Check sheet for the drawn part. Datum: minimum x, y, z corner. Units: mm. Coordinates: 2 decimals unless noted, no trailing zeros. Write each loop counter-clockwise with the first axis right and the second up, starting at its lowest first coordinate (ties: lowest second). Pieces come first, ordered by that corner, then holes. Notation, with made-up numbers: (20, 13) -> (50, 13) arc R28 ccw to (50, 50) -> close; hole circle Ø8 at (2, 29.5). An arc over 180 degrees is marked (long way). Answer in a Markdown table with one row per item. Add a question column.
1. Scan lines: L1, parallel to X at y = 1.05, z = 3.1; L2, parallel to Z at x = 54.9, y = 1.45; L3, parallel to X at y = 1.75, z = 29. Record each from-to range of solid material in increasing order. Write a range as from..to.
2. Cross-section at B-B on x = 54.9. Record the cut outline in (y, z), and give its area (3 significant figures).
3. Cross-section at A-A on z = 3.1. Record the cut outline in (x, y), and give its area (3 significant figures).
4. Cross-section at C-C on y = 1.3. Record the cut outline in (x, z).
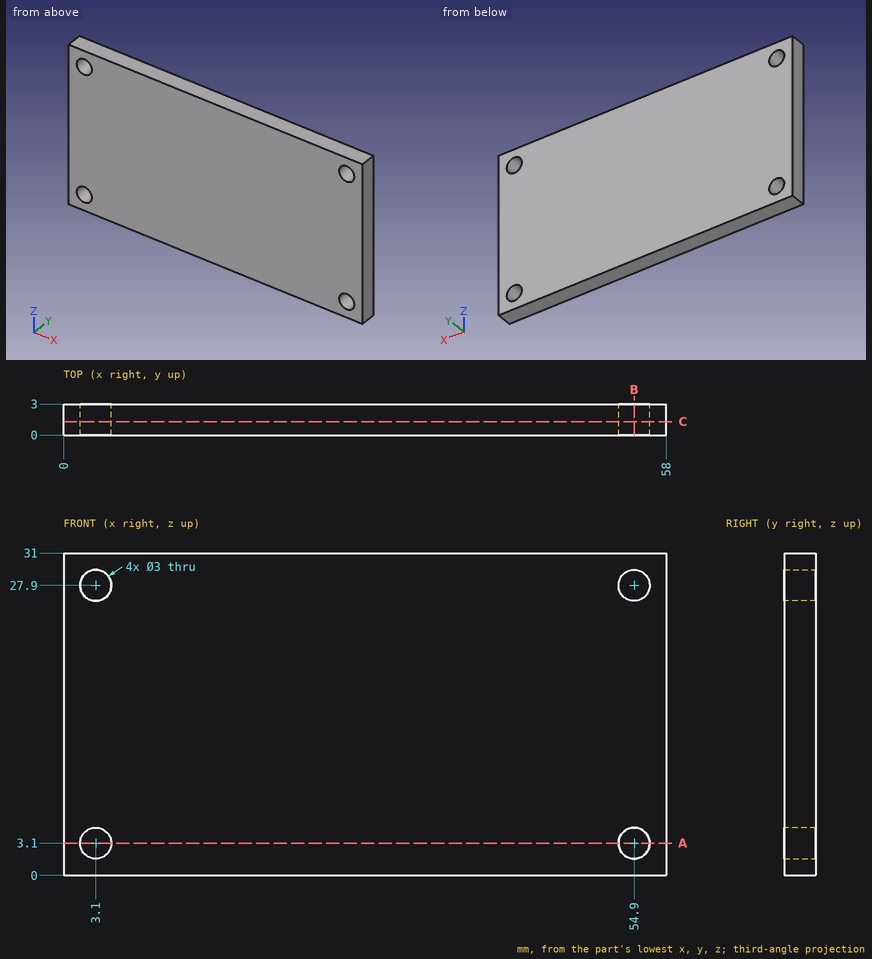
Results found:
| question | item | result |
|---|---|---|
| 1 | L1 | x = 0..1.6, 4.6..53.4, 56.4..58 |
| 1 | L2 | z = 0..1.6, 4.6..26.4, 29.4..31 |
| 1 | L3 | x = 0..2.08, 4.12..53.88, 55.92..58 |
| 2 | outline | (0, 0) -> (3, 0) -> (3, 1.6) -> (0, 1.6) -> close; (0, 4.6) -> (3, 4.6) -> (3, 26.4) -> (0, 26.4) -> close; (0, 29.4) -> (3, 29.4) -> (3, 31) -> (0, 31) -> close |
| 2 | area | 75.0 mm^2 |
| 3 | outline | (0, 0) -> (1.6, 0) -> (1.6, 3) -> (0, 3) -> close; (4.6, 0) -> (53.4, 0) -> (53.4, 3) -> (4.6, 3) -> close; (56.4, 0) -> (58, 0) -> (58, 3) -> (56.4, 3) -> close |
| 3 | area | 156 mm^2 |
| 4 | outline | (0, 0) -> (58, 0) -> (58, 31) -> (0, 31) -> close; hole circle Ø3 at (3.1, 3.1); hole circle Ø3 at (3.1, 27.9); hole circle Ø3 at (54.9, 3.1); hole circle Ø3 at (54.9, 27.9) |
